from build123d import *

# Parameters (mm, degrees)
F0_R     = 11.2
F1_DEPTH = 2
F2_R     = 6
F3_DEPTH = 1.5
F4_R     = 3.95
F5_DEPTH = 10
F6_R     = 1.99999


# Not quite as in the source:
# - a fillet or chamfer is up to 0.001 mm smaller than in the source, because OpenCascade refuses the exact size


with BuildPart() as f1:
    # F0 (on Top) → F1 (new body)
    with BuildSketch(Plane.XY):
        Circle(F0_R)
    extrude(amount=F1_DEPTH)

    # F2 (on face) → F3 (join)
    with BuildSketch(Plane.XY.offset(2)):
        Circle(F2_R)
    extrude(amount=F3_DEPTH)

    # F4 (on face) → F5 (join)
    with BuildSketch(Plane.XY.offset(3.5)):
        Circle(F4_R)
    extrude(amount=F5_DEPTH)

    # F6 (radius 2 in the source; OpenCascade refuses exactly that, so slightly less here)
    f6_edges = [f1.edges().sort_by_distance(p)[0] for p in [
        (-11.2, 0, 0),
    ]]
    fillet(f6_edges, radius=F6_R)


solid = f1.part
Check sheet for the modelled part. Datum: model origin and axes. Units: mm. A direction names the side the tool comes from. Give positions to 0.01 mm unless a question says otherwise; leave off trailing zeros. Write each loop counter-clockwise with the first axis right and the second up, starting at its lowest first coordinate (ties: lowest second). Pieces come first, ordered by that corner, then holes. Notation, with made-up numbers: (5.5, 11) -> (30.5, 11) arc R33 ccw to (30.5, 46) -> close; hole circle Ø5 at (60.5, -3.5). An arc over 180 degrees is marked (long way). One line per item, written item: value. Start each with the question number.
Item 1: Material ranges on probe 1 along Z at (x, y) = (2.25, -7); probe 2 along X at (y, z) = (0.5, 11); probe 3 along Y at (x, z) = (-10, 1), recorded low to high. Write a range as from..to.
Item 2: Gauge pin test, flat ends, axial feed: pin 1 (3 mm diameter, centred on x = 0, z = 11, fed in from +Y); pin 2 (8 mm diameter, centred on y = 6.5, z = 1.5, fed in from -X); pin 3 (5 mm diameter, centred on y = 3, z = 11, fed in from -X). Record the tip position at first contact, or that the pin passes through.
Item 3: Section check C-C on z = 4. Record the cut outline in (x, y), then the cut area to 3 significant figures.
Item 4: Tool access check on faces 1 (the flat face through (5, -5, 2)), 2 (the flat face through (0, 0, 13.5)). Record the directions out of +Z, -Z, +X, -X, +Y, -Y that give a thin tool (end or side, any length) a straight path to the whole face; none if there is none.
Results list:
1. probe 1: 0..2
1. probe 2: -3.92..3.92
1. probe 3: -4.42..4.42
2. pin 1: y = 3.95
2. pin 2: x = -10.91
2. pin 3: x = -3.92
3. outline: circle Ø7.9 at (0, 0)
3. area: 49.0 mm²
4. face 1: +Z
4. face 2: +Z, +X, -X, +Y, -Y
